Read the model definition and answer for the solid it produces. Units are mm, in the model's axes. Coordinates: 2 decimals unless noted, no trailing zeros. Order: outer loops, then holes, each group sorted by start corner. A loop starts at its lowest first (then second) coordinate and runs counter-clockwise, first axis right, second up. Notation, with made-up numbers: (-13, 79) - (36, 79) arc R28 cw to (36, 107) - close; hole circle Ø11 at (75.5, -5). An arc over 180 degrees is marked (long way). Use one line per item in the form item = value.
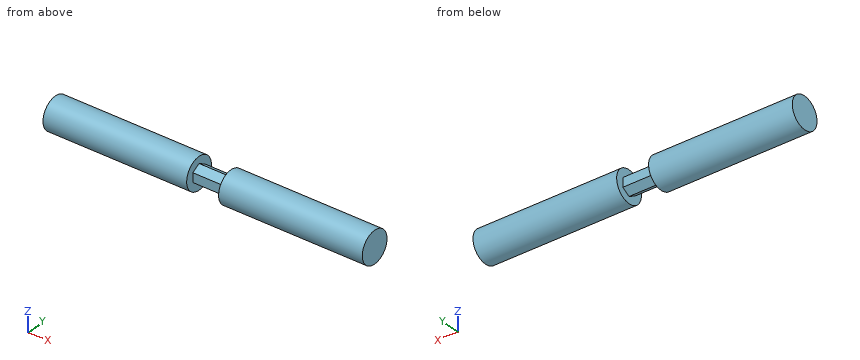
Autodesk Inventor part; units mm, degrees
ref_plane "YZ Plane" through (0, 0, 0) normal (1, 0, 0) x (0, 1, 0)
ref_plane "XZ Plane" through (0, 0, 0) normal (0, 1, 0) x (-1, 0, 0)
ref_plane "XY Plane" through (0, 0, 0) normal (0, 0, 1) x (1, 0, 0)
sketch "Sketch1" plane through (0, 0, 0) normal (1, 0, 0) x (0, 1, 0)
  circle A0 centre (0, 0) radius 12.7
  dimension "d0" = 25.4
extrude "Extrusion1" add sketch "Sketch1" against normal blind 254
sketch "Sketch2" plane through (0, 0, 0) normal (1, 0, 0) x (0, 0, -1)
  line L0 (3.6609, 6.353) -> (7.3323, 0.006)
  line L1 (7.3323, 0.006) -> (3.6714, -6.347)
  line L2 (3.6714, -6.347) -> (-3.6609, -6.353)
  line L3 (-3.6609, -6.353) -> (-7.3323, -0.006)
  line L4 (-7.3323, -0.006) -> (-3.6714, 6.347)
  line L5 (-3.6714, 6.347) -> (3.6609, 6.353)
  circle A0 centre (0, 0) radius 12.7
  dimension "d3" = 6.35
extrude "Extrusion2" cut sketch "Sketch2" against normal blind 254
extrude "Extrusion3" add sketch "Sketch2" against normal blind 114.3 contours L0 L1 L2 L3 L4 L5 | A0
sketch "Sketch3" plane through (-254, 0, 0) normal (-1, 0, 0) x (0, 0, 1)
  circle A0 centre (0, 0) radius 12.7
  circle A1 centre (0, 0) radius 12.7
extrude "Extrusion4" add sketch "Sketch3" against normal blind 114.3
properties part number "pin"
(1) Section C-C, the plane x = -57.5 is taken. Write down the section's boundary in (y, z), then the cut area to 3 significant figures.
Answer list:
outline = circle Ø25.4 at (0, 0)
area = 507 mm2
(2) Given pin 1 Ø6 at (x, z) = (-26.5, -4.5) entering from +Y; pin 2 Ø6 at (x, z) = (-193.5, 8.5) entering from +Y; pin 3 Ø1.5 at (x, y) = (-154.5, 3.5) entering from +Z, each flat-ended and moving along its own axis, determine where each tip first touches the part or whether it passes through.
Answer list:
pin_1 = 12.61
pin_2 = 11.45
pin_3 = 12.4
(3) Section B-B, the plane y = -9.5 is taken. Write down the section's boundary in (x, z).
Answer list:
outline = (-254, -8.43) - (-139.7, -8.43) - (-139.7, 8.43) - (-254, 8.43) - close; (-114.3, -8.43) - (0, -8.43) - (0, 8.43) - (-114.3, 8.43) - close
(4) Straight lines are drawn through the part: L1, parallel to X at y = -3.75, z = 6.5; L2, parallel to Z at x = -232, y = -0.5; L3, parallel to Z at x = -144.5, y = -5. For each, find the intervals that lie inside material, in ascending order.
Answer list:
L1 = -254 to -139.7, -114.3 to 0
L2 = -12.69 to 12.69
L3 = -11.67 to 11.67
(5) Section A-A, the plane z = 0 is taken. Write down the section's boundary in (x, y), then the cut area to 3 significant figures.
Answer list:
outline = (-254, -12.7) - (-139.7, -12.7) - (-139.7, -6.35) - (-114.3, -6.35) - (-114.3, -12.7) - (0, -12.7) - (0, 12.7) - (-114.3, 12.7) - (-114.3, 6.35) - (-139.7, 6.35) - (-139.7, 12.7) - (-254, 12.7) - close
area = 6,130 mm2
